The listing builds one solid part. Answer for the finished solid, in the listing's coordinates (mm). Round coordinates to 2 decimals unless told otherwise and drop trailing zeros. Order: outer loops, then holes, each group sorted by start corner. A loop starts at its lowest first (then second) coordinate and runs counter-clockwise, first axis right, second up. Notation, with made-up numbers: (-0.5, 46) - (27.5, 46) arc R8 ccw to (27.5, 59) - close; hole circle Ø2 at (83.5, -31). An arc over 180 degrees is marked (long way). Write item = value, one per line.
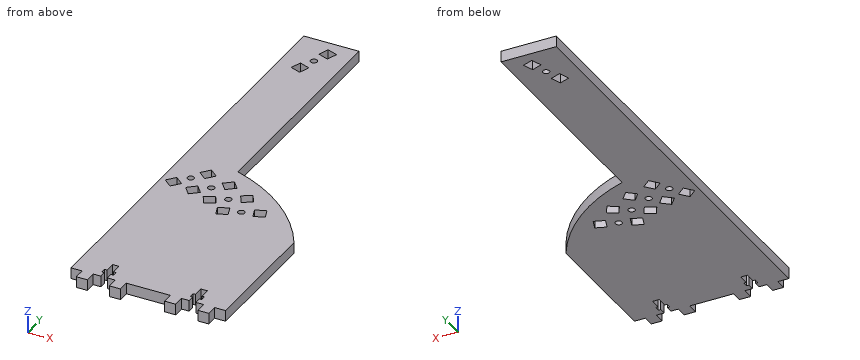
from build123d import *

# Parameters (mm, degrees)
ESQUISSE1_R        = 1.5
BOSS_EXTRU_1_DEPTH = 5


with BuildPart() as part:
    # Esquisse1 → Boss.-Extru.1 (new body)
    with BuildSketch(Plane.XY):
        with BuildLine():
            Line((-21.5, 0), (-25, 0))
            Line((-25, 0), (-25, -5))
            Line((-25, -5), (-30, -5))
            Line((-30, -5), (-30, 0))
            Line((-30, 0), (-35, 0))
            Line((-35, 0), (-35, 200))
            Line((-35, 200), (-10, 200))
            Line((-10, 200), (-10, 95.993420768))
            ThreePointArc((-10, 95.993420768), (16.02346259, 81.616607057), (35, 58.729833462))
            Line((35, 58.729833462), (35, 0))
            Line((35, 0), (30, 0))
            Line((30, 0), (30, -5))
            Line((30, -5), (25, -5))
            Line((25, -5), (25, 0))
            Line((25, 0), (21.5, 0))
            Line((21.5, 0), (21.5, 3))
            Line((21.5, 3), (22.6, 3))
            Line((22.6, 3), (22.6, 5.3))
            Line((22.6, 5.3), (21.5, 5.3))
            Line((21.5, 5.3), (21.5, 10))
            Line((21.5, 10), (18.5, 10))
            Line((18.5, 10), (18.5, 5.3))
            Line((18.5, 5.3), (17.4, 5.3))
            Line((17.4, 5.3), (17.4, 3))
            Line((17.4, 3), (18.5, 3))
            Line((18.5, 3), (18.5, 0))
            Line((18.5, 0), (15, 0))
            Line((15, 0), (15, -5))
            Line((15, -5), (10, -5))
            Line((10, -5), (10, 0))
            Line((10, 0), (-10, 0))
            Line((-10, 0), (-10, -5))
            Line((-10, -5), (-15, -5))
            Line((-15, -5), (-15, 0))
            Line((-15, 0), (-18.5, 0))
            Line((-18.5, 0), (-18.5, 3))
            Line((-18.5, 3), (-17.4, 3))
            Line((-17.4, 3), (-17.4, 5.3))
            Line((-17.4, 5.3), (-18.5, 5.3))
            Line((-18.5, 5.3), (-18.5, 10))
            Line((-18.5, 10), (-21.5, 10))
            Line((-21.5, 10), (-21.5, 5.3))
            Line((-21.5, 5.3), (-22.6, 5.3))
            Line((-22.6, 5.3), (-22.6, 3))
            Line((-22.6, 3), (-21.5, 3))
            Line((-21.5, 3), (-21.5, 0))
        make_face()
        with Locations((-24.543125869, 83.023041686)):
            Circle(ESQUISSE1_R, mode=Mode.SUBTRACT)
        with Locations((-13.758152943, 80.249762934)):
            Circle(ESQUISSE1_R, mode=Mode.SUBTRACT)
        with Locations((-3.618602792, 75.645825623)):
            Circle(ESQUISSE1_R, mode=Mode.SUBTRACT)
        with Locations((5.567439485, 69.351118058)):
            Circle(ESQUISSE1_R, mode=Mode.SUBTRACT)
        with Locations((-22.5, 185)):
            Circle(ESQUISSE1_R, mode=Mode.SUBTRACT)
        Polygon((-29.672175025, 80.799788495), (-32.886113073, 76.969566279), (-29.055890858, 73.755628231), (-25.841952809, 77.585850447), align=None, mode=Mode.SUBTRACT)
        Polygon((-23.244298928, 88.460232926), (-20.03036088, 92.290455142), (-16.200138664, 89.076517093), (-19.414076712, 85.246294878), align=None, mode=Mode.SUBTRACT)
        Polygon((-19.195344183, 78.950935993), (-23.025566399, 75.736997945), (-19.81162835, 71.906775729), (-15.981406135, 75.120713778), align=None, mode=Mode.SUBTRACT)
        Polygon((-11.534899752, 85.37881209), (-7.704677536, 88.592750139), (-4.490739488, 84.762527923), (-8.320961703, 81.548589875), align=None, mode=Mode.SUBTRACT)
        Polygon((-9.198729811, 75.310889132), (-13.52885683, 72.810889132), (-11.02885683, 68.480762114), (-6.698729811, 70.980762114), align=None, mode=Mode.SUBTRACT)
        Polygon((-0.538475773, 80.310889132), (3.791651246, 82.810889132), (6.291651246, 78.480762114), (1.961524227, 75.980762114), align=None, mode=Mode.SUBTRACT)
        Polygon((0.013926023, 69.990248894), (-4.684537081, 68.280148177), (-2.974436364, 63.581685073), (1.72402674, 65.29178579), align=None, mode=Mode.SUBTRACT)
        Polygon((9.410852231, 73.410450327), (14.109315335, 75.120551044), (15.819416051, 70.42208794), (11.120952947, 68.711987223), align=None, mode=Mode.SUBTRACT)
        Polygon((-26.559332269, 181.156587254), (-28.269432985, 176.45812415), (-23.570969881, 174.748023434), (-21.860869165, 179.446486538), align=None, mode=Mode.SUBTRACT)
        Polygon((-23.139130835, 190.553513462), (-21.429030119, 195.251976566), (-16.730567015, 193.54187585), (-18.440667731, 188.843412746), align=None, mode=Mode.SUBTRACT)
    extrude(amount=BOSS_EXTRU_1_DEPTH)


solid = part.part
Q1. Section B-B on z = 2.5 is taken. Count the separate pieces of the cut face and the enclosed holes in it, then the cut area to 3 significant figures.
Model answer:
separate_pieces = 1
enclosed_holes = 15
area = 8,440 mm^2
Q2. Section A-A on y = 166.5 is taken. Determine the outline of the cut face in (x, z).
Model answer:
outline = (-35, 0) - (-10, 0) - (-10, 5) - (-35, 5) - close
Q3. Find the intervals of material crossed by line 1 (X direction, y = 7.5, z = 1.15); line 2 (X direction, y = 85.5, z = 0.65); line 3 (X direction, y = 185, z = 1.75), in increasing order. Write a range as from..to.
Model answer:
line_1 = -35..-21.5, -18.5..18.5, 21.5..35
line_2 = -35..-19.72, -19.2..-11.39, -5.11..10.93
line_3 = -35..-24, -21..-10
Q4. Flat-ended cylindrical pins translate along their axes: P1, Ø0.6, axis at x = 18, z = 3, coming from the -Y side; P2, Ø0.9, axis at x = -19.5, z = 1.5, coming from the -Y side; P3, Ø2, axis at y = 163, z = 4.5, coming from the +X side. Find the tip coordinate at first contact, or state that the pin passes through.
Model answer:
P1 = 0
P2 = 10
P3 = -10
